Source: CAD feature listing. Evaluate the final solid. Frame: model axes, mm. A direction names the side the tool comes from. Give positions to 0.01 mm unless a question says otherwise; leave off trailing zeros. Order: outer loops, then holes, each group sorted by start corner. A loop starts at its lowest first (then second) coordinate and runs counter-clockwise, first axis right, second up.
```python
from build123d import *

# Parameters (mm, degrees)
ESQUISSE1_W             = 80
ESQUISSE1_H             = 100
BOSS_EXTRU_1_DEPTH      = 10
ENL_V_START             = -10
ENL_V_MAT_EXTRU_2_DEPTH = 10


# Read off the part's stored shape, not the designer's step: Enlèv. mat.-Extru.2
with BuildPart() as part:
    # Esquisse1 → Boss.-Extru.1 (new body)
    with BuildSketch(Plane.XY):
        Rectangle(ESQUISSE1_W, ESQUISSE1_H)
    extrude(amount=BOSS_EXTRU_1_DEPTH)

    # Enlèv. mat.-Extru.2 outline → Enlèv. mat.-Extru.2 (cut)
    with BuildSketch(Plane.XY.offset(10).offset(ENL_V_START)):
        Polygon((-40, -50), (-10, -50), (-10, -30), (-27, -24.083920217), (-38, -7.380627128), (-38, 15.619372872), (-32, 34.6981569), (-23.773026842, 42), (-28, 32.937290807), (-34, 13.858506778), (-34, -6.141493222), (-12.5, -18.898844044), (12.5, -18.898844044), (34, -6.141493222), (34, 13.858506778), (28, 32.937290807), (23.773026842, 42), (32, 34.6981569), (38, 15.619372872), (38, -7.380627128), (27, -24.083920217), (10, -30), (10, -50), (40, -50), (40, 50), (-40, 50), align=None)
    extrude(amount=ENL_V_MAT_EXTRU_2_DEPTH, mode=Mode.SUBTRACT)


solid = part.part
```
1) Section query B-B, the plane y = 36.5. Return the cut outline in (x, z), and give its area (3 significant figures).
Report:
outline: (-29.97, 0) - (-26.34, 0) - (-26.34, 10) - (-29.97, 10) - close; (26.34, 0) - (29.97, 0) - (29.97, 10) - (26.34, 10) - close
area: 72.6 mm2
2) Draft query along Y for faces 4 (the flat face through (0, -18.899, 5)), 5 (the flat face through (-25.86, 37.53, 4.93)), 6 (the flat face through (0, -21, 10)). Return one class per face: +Y half, -Y half, draft (parallel to the pull), parting line (faces both ways), or undercut.
Report:
face 4: +Y half
face 5: undercut
face 6: draft
3) Pin query (flat end, axial travel): pin 1 (4 mm diameter, centred on x = 17.5, z = 3, fed in from -Y); pin 2 (6 mm diameter, centred on x = -14, z = 7.5, fed in from +Y); pin 3 (3 mm diameter, centred on y = -44.5, z = 5, fed in from -X). Return the tip coordinate at first contact, or that it passes through.
Report:
pin 1: stops at y = -28.09
pin 2: stops at y = -16.23
pin 3: stops at x = -10
4) Reachability of faces 1 (the flat face through (-30.96, 23.53, 4.93)), 2 (the flat face through (-10, -40, 5)), 3 (the flat face through (10, -40, 5)) from +Z, -Z, +X, -X, +Y, -Y: full face, straight path, thin tool, end or side. Return the list, or none.
Report:
face 1: +Z, -Z
face 2: +Z, -Z, -X, -Y
face 3: +Z, -Z, +X, -Y
5) Section query C-C, the plane z = 7.5. Return the cut outline in (x, y).
Report:
outline: (-38, -7.38) - (-27, -24.08) - (-10, -30) - (-10, -50) - (10, -50) - (10, -30) - (27, -24.08) - (38, -7.38) - (38, 15.62) - (32, 34.7) - (23.77, 42) - (28, 32.94) - (34, 13.86) - (34, -6.14) - (12.5, -18.9) - (-12.5, -18.9) - (-34, -6.14) - (-34, 13.86) - (-28, 32.94) - (-23.77, 42) - (-32, 34.7) - (-38, 15.62) - close
6) Section query A-A, the plane x = 33. Return the cut outline in (y, z), and give its area (3 significant figures).
Report:
outline: (-14.97, 0) - (-6.73, 0) - (-6.73, 10) - (-14.97, 10) - close; (17.04, 0) - (31.52, 0) - (31.52, 10) - (17.04, 10) - close
area: 227 mm2
7) Material intervals for L1, parallel to X at y = 13.5, z = 5; L2, parallel to X at y = -37, z = 6.75; L3, parallel to X at y = 28, z = 3.25, sorted ascending.
Report:
L1: x = -38 to -34, 34 to 38
L2: x = -10 to 10
L3: x = -34.11 to -29.55, 29.55 to 34.11
8) Section query D-D, the plane x = 4. Return the cut outline in (y, z), and give its area (3 significant figures).
Report:
outline: (-50, 0) - (-18.9, 0) - (-18.9, 10) - (-50, 10) - close
area: 311 mm2
